Could you check a few things on this model? Use its own coordinates, in mm. Give positions to 0.01 mm unless a question says otherwise; leave off trailing zeros. Order: outer loops, then holes, each group sorted by start corner. A loop starts at its lowest first (then second) coordinate and runs counter-clockwise, first axis right, second up. Notation, with made-up numbers: M 85.5,37 L 98.5,37 A22 ccw 98.5,57 Z; hole C 25,3.5 d9. An arc over 180 degrees is marked long. Use a Markdown table: item, result. Add a question column.
```python
from build123d import *

# Parameters (mm, degrees)
SKETCH5_R           = 48.26
SKETCH5_R_2         = 2.15265
SKETCH5_R_3         = 3.5
SKETCH5_R_4         = 17.5
BOSS_EXTRUDE3_DEPTH = 3.175


with BuildPart() as part:
    # Sketch5 → Boss-Extrude3 (new body)
    with BuildSketch(Plane(origin=(0, 0, 0), x_dir=(0, 0, -1), z_dir=(1, 0, 0))):
        Circle(SKETCH5_R)
        with Locations((0, 45.085)):
            Circle(SKETCH5_R_2, mode=Mode.SUBTRACT)
        with Locations((-24.023795501, -9.950801949)):
            Circle(SKETCH5_R_3, mode=Mode.SUBTRACT)
        with Locations((31.87990923, 31.87990923)):
            Circle(SKETCH5_R_2, mode=Mode.SUBTRACT)
        with Locations((45.085, 0)):
            Circle(SKETCH5_R_2, mode=Mode.SUBTRACT)
        with Locations((24.018239985, 9.948012748)):
            Circle(SKETCH5_R_3, mode=Mode.SUBTRACT)
        with Locations((-9.9503853, 24.023968076)):
            Circle(SKETCH5_R_3, mode=Mode.SUBTRACT)
        with Locations((31.87990923, -31.87990923)):
            Circle(SKETCH5_R_2, mode=Mode.SUBTRACT)
        with Locations((0, -45.085)):
            Circle(SKETCH5_R_2, mode=Mode.SUBTRACT)
        with Locations((-31.87990923, -31.87990923)):
            Circle(SKETCH5_R_2, mode=Mode.SUBTRACT)
        with Locations((-45.085, 0)):
            Circle(SKETCH5_R_2, mode=Mode.SUBTRACT)
        with Locations((-31.87990923, 31.87990923)):
            Circle(SKETCH5_R_2, mode=Mode.SUBTRACT)
        Circle(SKETCH5_R_4, mode=Mode.SUBTRACT)
        with BuildLine():
            Line((20.434868218, -10.637719077), (33.719928863, -17.553483913))
            ThreePointArc((33.719928863, -17.553483913), (34.993654696, -19.123916601), (34.716893211, -21.126924191))
            ThreePointArc((34.716893211, -21.126924191), (13.899698625, -38.189108109), (-13.014558026, -38.49975168))
            ThreePointArc((-13.014558026, -38.49975168), (-14.514078084, -37.143257699), (-14.547802162, -35.121501281))
            Line((-14.547802162, -35.121501281), (-8.816223227, -21.284245682))
            ThreePointArc((-8.816223227, -21.284245682), (-7.568898247, -19.966485263), (-5.760575328, -19.817219233))
            ThreePointArc((-5.760575328, -19.817219233), (7.058440708, -19.392906461), (17.1511197, -11.478044227))
            ThreePointArc((17.1511197, -11.478044227), (18.632321778, -10.430021072), (20.434868218, -10.637719077))
        make_face(mode=Mode.SUBTRACT)
    extrude(amount=BOSS_EXTRUDE3_DEPTH)


solid = part.part
```
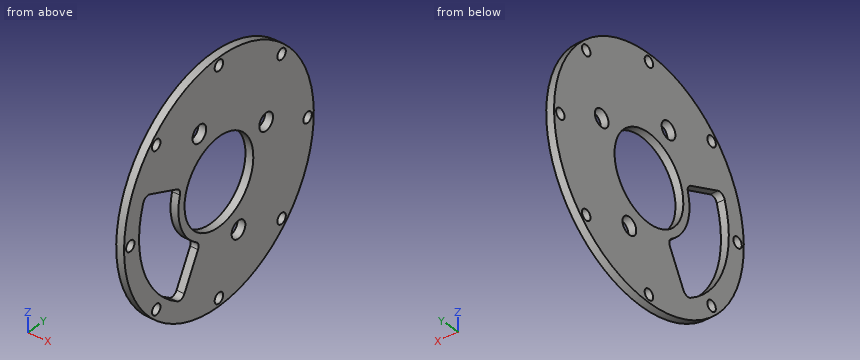
1) For pin 1 (3.5 mm diameter, centred on y = 0, z = -45.085, fed in from -X); pin 2 (1.5 mm diameter, centred on x = 3, y = 4.5, fed in from +Z); pin 3 (1 mm diameter, centred on x = 0.5, z = -15.5, fed in from +Y); pin 4 (1 mm diameter, centred on x = 1.5, z = -1.5, fed in from +Y), each with a flat end and sliding along its axis, tell me the tip position at first contact or that it passes through.
2) Suppose I cut it at A-A on y = 0. Please give me the cut outline in (x, z) (3 decimals).
3) Suppose I cut it at C-C on y = -25. Please give me the cut outline in (x, z) (3 decimals).
4) Please list where these lines run through material, in increasing order: line 1 (Y direction, x = 0.85, z = 0); line 2 (Z direction, x = 1, y = 32); line 3 (Y direction, x = 1.45, z = -27). Write a range as from..to.
5) Suppose I cut it at D-D on z = 0. Please give me the cut outline in (x, y) (1 decimal).
6) Suppose I cut it at B-B on z = -10.5. Please give me the cut outline in (x, y) (3 decimals), and give its area (3 significant figures).
Values found:
| question | item | result |
|---|---|---|
| 1 | pin 1 | passes through |
| 1 | pin 2 | stops at z = 48.11 |
| 1 | pin 3 | stops at y = 45.87 |
| 1 | pin 4 | stops at y = 48.25 |
| 2 | outline | M 0,-48.26 L 3.175,-48.26 L 3.175,-47.238 L 0,-47.238 Z; M 0,-42.932 L 3.175,-42.932 L 3.175,-17.5 L 0,-17.5 Z; M 0,17.5 L 3.175,17.5 L 3.175,42.932 L 0,42.932 Z; M 0,47.238 L 3.175,47.238 L 3.175,48.26 L 0,48.26 Z |
| 3 | outline | M 0,-41.28 L 3.175,-41.28 L 3.175,-32.041 L 0,-32.041 Z; M 0,10.355 L 3.175,10.355 L 3.175,41.28 L 0,41.28 Z |
| 4 | line 1 | y = -48.26..-47.24, -42.93..-40.64, -20.64..-17.5, 17.5..42.93, 47.24..48.26 |
| 4 | line 2 | z = -36.13..-34.03, -29.73..29.73, 34.03..36.13 |
| 4 | line 3 | y = -40..-30.37, -14.06..8.12, 11.78..40 |
| 5 | outline | M 0,-48.3 L 3.2,-48.3 L 3.2,-47.2 L 0,-47.2 Z; M 0,-42.9 L 3.2,-42.9 L 3.2,-40.6 L 0,-40.6 Z; M 0,-20.6 L 3.2,-20.6 L 3.2,-17.5 L 0,-17.5 Z; M 0,17.5 L 3.2,17.5 L 3.2,42.9 L 0,42.9 Z; M 0,47.2 L 3.2,47.2 L 3.2,48.3 L 0,48.3 Z |
| 6 | outline | M 0,-47.104 L 3.175,-47.104 L 3.175,-39.26 L 0,-39.26 Z; M 0,-17.767 L 3.175,-17.767 L 3.175,-14 L 0,-14 Z; M 0,14 L 3.175,14 L 3.175,47.104 L 0,47.104 Z |
| 6 | area | 142 mm^2 |
